For this review, take the finished solid that the model builds, in its own axes (mm). Face numbers are marked on the shaded views. A direction names the side the tool comes from. Give positions to 0.01 mm unless a question says otherwise; leave off trailing zeros. Write each loop counter-clockwise with the first axis right and the second up, starting at its lowest first coordinate (ties: lowest second). Pieces come first, ordered by that corner, then holes. Notation, with made-up numbers: M 60.5,16 L 69.5,16 A33 ccw 69.5,47 Z; hole C 22,38 d8. An arc over 180 degrees is marked long. Use one line per item in the form item = value. Start each with the question number.
Q1. For probe 1 along Y at (x, z) = (25.4, 4); probe 2 along Z at (x, y) = (4.5, 12.5); probe 3 along Z at (x, y) = (53, 11.25), list the stretches that pass through material, from the lowest coordinate up. Write a range as [from, to].
Q2. Consider section D-D on x = 4. Write out the cut boundary in (y, z) (3 decimals).
Q3. Clearance check with flat-ended pins moving along their axes: pin 1 Ø2 at (x, y) = (11, 9) entering from +Z; pin 2 Ø12 at (y, z) = (8, 38) entering from -X; pin 3 Ø12 at (y, z) = (4, 34) entering from +X; pin 4 Ø3 at (x, y) = (34.5, 7) entering from +Z. State where each tip first meets the part, or that it passes through.
Q4. Consider section C-C on y = 9.75. Write out the cut boundary in (x, z), and give its area (3 significant figures).
Q5. Consider section A-A on x = 25.4. Write out the cut boundary in (y, z), and give its area (3 significant figures).
Q6. Tool access review of the marked faces 4, 5 and 6: name each direction out of +Z, -Z, +X, -X, +Y, -Y from which nothing blocks a thin tool from reaching the whole face with its end or side.
Q7. Consider section B-B on z = 4.5. Write out the cut boundary in (x, y).
Q8. Mouldability with a two-part tool opening along X and no side actions: class the marked faces 1, 2 and 3 as released by +X, released by -X, zero draft, split by the parting line, or undercut.
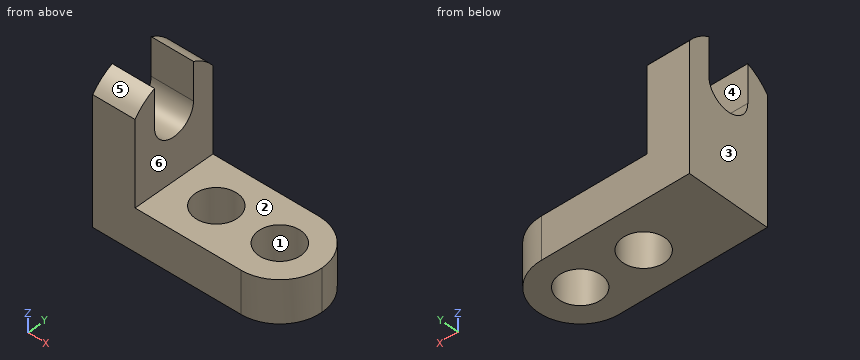
```python
from build123d import *

# Parameters (mm, degrees)
F0_W      = 63.5
F0_H      = 44.45
F1_DEPTH  = 25.4
F2_DEPTH  = 6.35
F3_W      = 44.45
F3_H      = 31.75
F4_DEPTH  = 25.4
F5_R      = 6.35
F6_DEPTH  = 25.4
F8_DEPTH  = 25.4
F10_DEPTH = 25.4


with BuildPart() as f1:
    # F0 (on Front) → F1 (new body)
    with BuildSketch(Plane.XZ):
        with Locations((31.75, 22.225)):
            Rectangle(F0_W, F0_H)
    extrude(amount=-F1_DEPTH)

    # F2 (cut): a face of the model
    f2_faces = [f1.faces().sort_by_distance(p)[0] for p in [
        (63.5, 12.7, 22.225),
    ]]
    extrude(f2_faces, amount=-F2_DEPTH, mode=Mode.SUBTRACT)

    # F3 (on face) → F4 (cut)
    with BuildSketch(Plane.XZ):
        with Locations((34.925, 28.575)):
            Rectangle(F3_W, F3_H)
    extrude(amount=-F4_DEPTH, mode=Mode.SUBTRACT)

    # F5 (on face) → F6 (cut)
    with BuildSketch(Plane.XY.offset(12.7)):
        with Locations((25.4, 12.7)):
            Circle(F5_R)
        with Locations((44.45, 12.7)):
            Circle(F5_R)
    extrude(amount=-F6_DEPTH, mode=Mode.SUBTRACT)

    # F7 (on face) → F8 (cut)
    with BuildSketch(Plane.XY.offset(12.7)):
        with BuildLine():
            ThreePointArc((44.45, 25.4), (53.4302561211, 21.6802561211), (57.15, 12.7))
            Line((57.15, 12.7), (57.15, 25.4))
            Line((57.15, 25.4), (44.45, 25.4))
        make_face()
        with BuildLine():
            ThreePointArc((57.15, 12.7), (53.4302561211, 3.7197438789), (44.45, 0))
            Line((44.45, 0), (57.15, 0))
            Line((57.15, 0), (57.15, 12.7))
        make_face()
    extrude(amount=-F8_DEPTH, mode=Mode.SUBTRACT)

    # F9 (on face) → F10 (cut)
    with BuildSketch(Plane.YZ.offset(12.7)):
        with BuildLine():
            ThreePointArc((12.7, 44.45), (15.9434155936, 44.1151377178), (19.05, 43.1246778315))
            Line((19.05, 43.1246778315), (19.05, 44.45))
            Line((19.05, 44.45), (12.7, 44.45))
        make_face()
        with BuildLine():
            Line((6.35, 44.45), (6.35, 43.1246778315))
            ThreePointArc((6.35, 43.1246778315), (9.4565844064, 44.1151377178), (12.7, 44.45))
            Line((12.7, 44.45), (6.35, 44.45))
        make_face()
        with BuildLine():
            ThreePointArc((0, 38.1), (2.8492400381, 41.0240221774), (6.35, 43.1246778315))
            Line((6.35, 43.1246778315), (6.35, 44.45))
            Line((6.35, 44.45), (0, 44.45))
            Line((0, 44.45), (0, 38.1))
        make_face()
        with BuildLine():
            ThreePointArc((6.35, 31.75), (12.7, 25.4), (19.05, 31.75))
            ThreePointArc((19.05, 31.75), (12.7, 38.1), (6.35, 31.75))
        make_face()
        with BuildLine():
            ThreePointArc((6.35, 31.75), (12.7, 38.1), (19.05, 31.75))
            Line((19.05, 31.75), (19.05, 43.1246778315))
            ThreePointArc((19.05, 43.1246778315), (15.9434155936, 44.1151377178), (12.7, 44.45))
            ThreePointArc((12.7, 44.45), (9.4565844064, 44.1151377178), (6.35, 43.1246778315))
            Line((6.35, 43.1246778315), (6.35, 31.75))
        make_face()
        with BuildLine():
            Line((19.05, 44.45), (19.05, 43.1246778315))
            ThreePointArc((19.05, 43.1246778315), (22.5507599619, 41.0240221774), (25.4, 38.1))
            Line((25.4, 38.1), (25.4, 44.45))
            Line((25.4, 44.45), (19.05, 44.45))
        make_face()
    extrude(amount=-F10_DEPTH, mode=Mode.SUBTRACT)


solid = f1.part
```
Working result:
q1.probe_1 = [0, 6.35], [19.05, 25.4]
q1.probe_2 = [0, 25.4]
q1.probe_3 = [0, 12.7]
q2.outline = M 0,0 L 25.4,0 L 25.4,38.1 A15.875 ccw 19.05,43.125 L 19.05,31.75 A6.35 cw 6.35,31.75 L 6.35,43.125 A15.875 ccw 0,38.1 Z
q3.pin_1 = 27.48
q3.pin_2 = 0
q3.pin_3 = 12.7
q3.pin_4 = 12.7
q4.outline = M 0,0 L 19.78,0 L 19.78,12.7 L 12.7,12.7 L 12.7,26.13 L 0,26.13 Z; M 31.02,0 L 38.83,0 L 38.83,12.7 L 31.02,12.7 Z; M 50.07,0 L 56.8,0 L 56.8,12.7 L 50.07,12.7 Z
q4.area = 606 mm²
q5.outline = M 0,0 L 6.35,0 L 6.35,12.7 L 0,12.7 Z; M 19.05,0 L 25.4,0 L 25.4,12.7 L 19.05,12.7 Z
q5.area = 161 mm²
q6.face_4 = +Z, +X, -X
q6.face_5 = +Z, +X, -X, -Y
q6.face_6 = +Z, +X, +Y, -Y
q7.outline = M 0,0 L 44.45,0 A12.7 ccw 44.45,25.4 L 0,25.4 Z; hole C 25.4,12.7 d12.7; hole C 44.45,12.7 d12.7
q8.face_1 = undercut
q8.face_2 = zero draft
q8.face_3 = released by -X
